from build123d import *

# Parameters (mm, degrees)
EXTRUDE001_DEPTH                     = 44
EXTRUDE001_ONTO_SKETCH001_ROLL_ANGLE = 90
SKETCH_R                             = 1.8
EXTRUDE_DEPTH                        = 2
CHAMFER_SIZE                         = 2


with BuildPart() as extrude001:
    # Sketch001 as drawn → Extrude001 (new)
    with BuildSketch(Plane.XY):
        Polygon((-20.25, 0), (20.25, 0), (20.25, -7), (16, -7), (16, -3), (-16, -3), (-16, -7), (-20.25, -7), align=None)
    extrude(amount=-EXTRUDE001_DEPTH)


with BuildPart() as extrude001_1:
    # Extrude001 onto Sketch001 roll: moved
    add(extrude001.part.rotate(Axis((0, 0, 0), (1, 0, 0)), EXTRUDE001_ONTO_SKETCH001_ROLL_ANGLE))


with BuildPart() as extrude001_2:
    # Extrude001 onto Sketch001 placement: moved
    add(extrude001_1.part)


with BuildPart() as chamfer_body:
    # Sketch → Extrude (new body)
    with BuildSketch(Plane.XY):
        with BuildLine():
            Line((-20.25, 44), (-20.25, 22))
            Line((-20.25, 22), (-27.25, 22))
            ThreePointArc((-27.25, 22), (-30.769759, 17), (-27.25, 12))
            Line((-27.25, 12), (-20.25, 12))
            Line((-20.25, 12), (-20.25, 0))
            Line((-20.25, 0), (20.25, 0))
            Line((20.25, 0), (20.25, 12))
            Line((20.25, 12), (27.25, 12))
            ThreePointArc((27.25, 12), (30.769759, 17), (27.25, 22))
            Line((27.25, 22), (20.25, 22))
            Line((20.25, 22), (20.25, 44))
            Line((20.25, 44), (-20.25, 44))
        make_face()
        with Locations((-25.4585, 17)):
            Circle(SKETCH_R, mode=Mode.SUBTRACT)
        with Locations((25.4585, 17)):
            Circle(SKETCH_R, mode=Mode.SUBTRACT)
    extrude(amount=EXTRUDE_DEPTH)

    # Fusion: union Extrude001
    add(extrude001_2.part)

    # Chamfer
    chamfer_edges = [chamfer_body.edges().sort_by_distance(p)[0] for p in [
        (-16, 22, -3),
        (16, 22, -3),
    ]]
    chamfer(chamfer_edges, length=CHAMFER_SIZE)


solid = chamfer_body.part
Part model, mm, in its own coordinate system. A direction names the side the tool comes from. Round coordinates to 2 decimals unless told otherwise and drop trailing zeros. Loops run counter-clockwise (first coordinate to the right, second up) from the corner with the lowest first, then second, coordinate; pieces in that order, holes last. Notation, with made-up numbers: (27.25, -17) - (31.25, -17) arc R8 ccw to (31.25, -2) - close; hole circle Ø5 at (-11, 56.5). An arc over 180 degrees is marked (long way). Answer as a JSON object with one key per item and string values.
Item 1: Band-saw the part on B-B on y = 17. List the corners of the cut face in (x, z), plus the area to 3 significant figures.
Output:
{"outline": "(-30.77, 0) - (-27.26, 0) - (-27.26, 2) - (-30.77, 2) - close; (-23.66, 0) - (-20.25, 0) - (-20.25, -7) - (-16, -7) - (-16, -5) - (-14, -3) - (14, -3) - (16, -5) - (16, -7) - (20.25, -7) - (20.25, 0) - (23.66, 0) - (23.66, 2) - (-23.66, 2) - close; (27.26, 0) - (30.77, 0) - (30.77, 2) - (27.26, 2) - close", "area": "268 mm2"}
Item 2: Wall check: L1, parallel to X at y = 7, z = 1.5; L2, parallel to Z at x = 7, y = 8; L3, parallel to Z at x = 22, y = 14.5. Give the ranges that are in metal, low to high.
Output:
{"L1": "-20.25 to 20.25", "L2": "-3 to 2", "L3": "0 to 2"}
Item 3: Band-saw the part on A-A on z = -5.75. List the corners of the cut face in (x, y), plus the area to 3 significant figures.
Output:
{"outline": "(-20.25, 0) - (-16, 0) - (-16, 44) - (-20.25, 44) - close; (16, 0) - (20.25, 0) - (20.25, 44) - (16, 44) - close", "area": "374 mm2"}
Item 4: Pin check, flat tips, straight feed: pin 1 (2 mm diameter, centred on y = 18, z = -6, fed in from +X); pin 2 (8 mm diameter, centred on x = 27, y = 19.5, fed in from -Z); pin 3 (1 mm diameter, centred on x = -22.5, z = 1.5, fed in from +Y); pin 4 (3 mm diameter, centred on x = 25.46, y = 17, fed in from -Z). Stop position of each tip, or through.
Output:
{"pin 1": "x = 20.25", "pin 2": "z = 0", "pin 3": "y = 22", "pin 4": "through"}
Item 5: Band-saw the part on C-C on y = 23. List the corners of the cut face in (x, z), plus the area to 4 significant figures.
Output:
{"outline": "(-20.25, -7) - (-16, -7) - (-16, -5) - (-14, -3) - (14, -3) - (16, -5) - (16, -7) - (20.25, -7) - (20.25, 2) - (-20.25, 2) - close", "area": "240.5 mm2"}
Item 6: Band-saw the part on D-D on z = -2.25. List the corners of the cut face in (x, y).
Output:
{"outline": "(-20.25, 0) - (20.25, 0) - (20.25, 44) - (-20.25, 44) - close"}
Item 7: Pull direction X, two halves, no side cores. Call faces 4 (the face through (0, 22, -3)), 5 (the face through (24, 12, 1)), 6 (the face through (30.77, 16.91, 0.99)), 7 (the face through (16, 22, -6)): pulls with the +X half, pulls with the -X half, needs draft (parallel to the pull), parting line crosses it, or undercut.
Output:
{"face 4": "undercut", "face 5": "needs draft", "face 6": "pulls with the +X half", "face 7": "undercut"}
Item 8: Tool access for faces 1 (the face through (-23, 17, 0)), 2 (the face through (-15, 22, -4)), 3 (the face through (-24, 22, 1)): list every direction of +Z, -Z, +X, -X, +Y, -Y with a clear straight run to the whole face (end or side of a thin tool).
Output:
{"face 1": "-Z, -X, +Y, -Y", "face 2": "-Z, +Y, -Y", "face 3": "+Z, -Z, -X, +Y"}
